Part model, mm, in its own coordinate system. Face numbers are marked on the shaded views. A direction names the side the tool comes from. Give positions to 0.01 mm unless a question says otherwise; leave off trailing zeros. Write each loop counter-clockwise with the first axis right and the second up, starting at its lowest first coordinate (ties: lowest second). Pieces come first, ordered by that corner, then holes. Notation, with made-up numbers: M 2.5,66 L 58.5,66 A34 ccw 58.5,104 Z; hole C 48.5,-16.5 d4. An arc over 180 degrees is marked long. Use a Markdown table: item, result.
```python
from build123d import *
from build123d.topology import SkipClean

# Parameters (mm, degrees)
SKETCH1_R           = 1.1
BOSS_EXTRUDE1_DEPTH = 1.5
SKETCH2_R           = 2.5
BOSS_EXTRUDE2_DEPTH = 1
BOSS_EXTRUDE3_DEPTH = 4
BOSS_EXTRUDE4_START = 5
SKETCH4_W           = 6
SKETCH4_H           = 14
SKETCH4_R           = 1.1
BOSS_EXTRUDE4_DEPTH = 5
FILLET4_R           = 3
FILLET1_R           = 0.5
SKETCH5_R           = 1.75
CUT_EXTRUDE1_DEPTH  = 4
FILLET3_R           = 2


with BuildPart() as part:
    # Sketch1 → Boss-Extrude1 (new body)
    with BuildSketch(Plane.XY):
        with BuildLine():
            Line((-17, 7), (0, 7))
            ThreePointArc((0, 7), (7, 0), (0, -7))
            Line((0, -7), (-17, -7))
            Line((-17, -7), (-17, 7))
        make_face()
        with Locations((-14, 3.5)):
            Circle(SKETCH1_R, mode=Mode.SUBTRACT)
        with Locations(Location((-14, -3.5, 0), (0, 0, 180))):
            Circle(SKETCH1_R, mode=Mode.SUBTRACT)
    extrude(amount=BOSS_EXTRUDE1_DEPTH)

    # Sketch2 → Boss-Extrude2 (add)
    with BuildSketch(Plane(origin=(0, 0, 0), x_dir=(-1, 0, 0), z_dir=(0, 0, -1))):
        Circle(SKETCH2_R)
    extrude(amount=BOSS_EXTRUDE2_DEPTH)

    # Sketch3 → Boss-Extrude3 (add)
    with BuildSketch(Plane(origin=(0, 0, -1), x_dir=(-1, 0, 0), z_dir=(0, 0, -1))):
        with BuildLine():
            Line((1.13862177, 1.394109201), (1.13862177, -1.394109201))
            ThreePointArc((1.13862177, -1.394109201), (-1.8, 0), (1.13862177, 1.394109201))
        make_face()
    extrude(amount=BOSS_EXTRUDE3_DEPTH)

    # Sketch4 → Boss-Extrude4 (add)
    with SkipClean():  # the faces are left unmerged after this step: merging them gives an invalid solid
        with BuildSketch(Plane(origin=(0, 0, 0), x_dir=(-1, 0, 0), z_dir=(0, 0, -1)).offset(BOSS_EXTRUDE4_START)):
            with Locations((14, 0)):
                Rectangle(SKETCH4_W, SKETCH4_H)
            with Locations((14, 3.5)):
                Circle(SKETCH4_R, mode=Mode.SUBTRACT)
            with Locations((14, -3.5)):
                Circle(SKETCH4_R, mode=Mode.SUBTRACT)
        extrude(amount=-BOSS_EXTRUDE4_DEPTH)

    # Fillet4
    fillet4_edges = [part.edges().sort_by_distance(p)[0] for p in [
        (-17, -7, -2.5),
        (-17, 7, -2.5),
    ]]
    fillet(fillet4_edges, radius=FILLET4_R)

    # Fillet1
    fillet1_edges = [part.edges().sort_by_distance(p)[0] for p in [
        (7, 0, 1.5),
        (-17, 0, 1.5),
        (-7, -7, 1.5),
        (-16.121320344, -6.121320344, 1.5),
        (-16.121320344, 6.121320344, 1.5),
        (-7, 7, 1.5),
    ]]
    fillet(fillet1_edges, radius=FILLET1_R)

    # Sketch5 → Cut-Extrude1 (cut)
    with BuildSketch(Plane.XY.offset(1.5)):
        with Locations((-14, 3.5)):
            Circle(SKETCH5_R)
        with Locations((-14, -3.5)):
            Circle(SKETCH5_R)
    extrude(amount=-CUT_EXTRUDE1_DEPTH, mode=Mode.SUBTRACT)

    # Fillet3
    fillet3_edges = [part.edges().sort_by_distance(p)[0] for p in [
        (-11, 0, 0),
    ]]
    fillet(fillet3_edges, radius=FILLET3_R)


solid = part.part
```
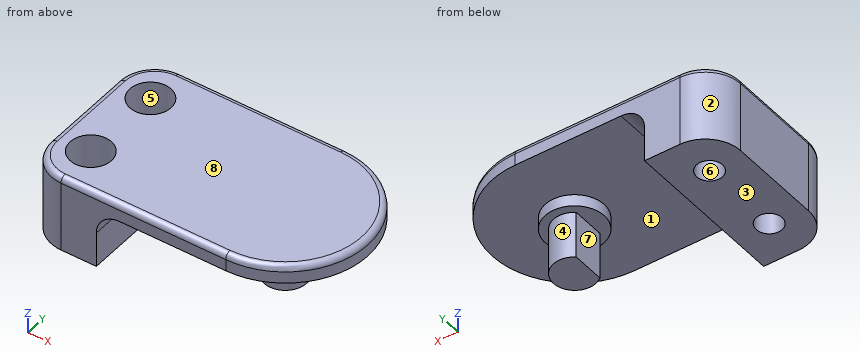
1. Cut at A-A, the plane z = -4. Give the cut face in (x, y), then the cut area to 3 significant figures.
Findings below:
| item | result |
|---|---|
| outline | M -17,-4 A3 ccw -14,-7 L -11,-7 L -11,7 L -14,7 A3 ccw -17,4 Z; M -1.14,-1.39 A1.8 ccw long -1.14,1.39 Z; hole C -14,-3.5 d2.2; hole C -14,3.5 d2.2 |
| area | 81.4 mm2 |
2. Drop flat-ended pins along their axis: P1, Ø2, axis at x = -4, z = -1.5, coming from the -Y side; P2, Ø1.5, axis at y = 3, z = -3.5, coming from the +X side; P3, Ø2.5, axis at x = -14, y = 3.5, coming from the +Z side; P4, Ø1.5, axis at y = 1, z = -2.5, coming from the +X side. Give the stop position or say it passes through.
Findings below:
| item | result |
|---|---|
| P1 | through |
| P2 | x = -11 |
| P3 | z = -2.5 |
| P4 | x = 1.78 |
3. Two-plate mould, pull along X, no slides. Class the marked faces 1, 2 and 3: released by +X, released by -X, zero draft, split by the parting line, or undercut.
Findings below:
| item | result |
|---|---|
| face 1 | undercut |
| face 2 | released by -X |
| face 3 | zero draft |
4. Drill centre lines: L1, parallel to Y at x = -14, z = -0.7; L2, parallel to Y at x = -14, z = -4; L3, parallel to X at y = -3, z = -4.5. Where is each one in solid material? Low to high.
Findings below:
| item | result |
|---|---|
| L1 | -7 to -5.25, -1.75 to 1.75, 5.25 to 7 |
| L2 | -7 to -4.6, -2.4 to 2.4, 4.6 to 7 |
| L3 | -17 to -14.98, -13.02 to -11 |
5. Tool access for the marked faces 4, 5, 6, 7 and 8: list every direction of +Z, -Z, +X, -X, +Y, -Y with a clear straight run to the whole face (end or side of a thin tool).
Findings below:
| item | result |
|---|---|
| face 4 | -Z |
| face 5 | +Z |
| face 6 | +Z, -Z |
| face 7 | -Z, +Y, -Y |
| face 8 | +Z, +X, -X, +Y, -Y |
6. Cut at B-B, the plane z = 0.25. Give the cut face in (x, y).
Findings below:
| item | result |
|---|---|
| outline | M -17,-4 A3 ccw -14,-7 L 0,-7 A7 ccw 0,7 L -14,7 A3 ccw -17,4 Z; hole C -14,-3.5 d3.5; hole C -14,3.5 d3.5 |
7. Cut at D-D, the plane z = -1.75. Give the cut face in (x, y).
Findings below:
| item | result |
|---|---|
| outline | M -17,-4 A3 ccw -14,-7 L -10.98,-7 L -10.98,7 L -14,7 A3 ccw -17,4 Z; M -1.14,-1.39 A1.8 ccw long -1.14,1.39 Z; hole C -14,-3.5 d3.5; hole C -14,3.5 d3.5 |
8. Cut at C-C, the plane y = 0. Give the cut face in (x, z), then the cut area to 3 significant figures.
Findings below:
| item | result |
|---|---|
| outline | M -17,-5 L -11,-5 L -11,-2 A2 cw -9,0 L -2.5,0 L -2.5,-1 L -1.14,-1 L -1.14,-5 L 1.8,-5 L 1.8,-1 L 2.5,-1 L 2.5,0 L 7,0 L 7,1 A0.5 ccw 6.5,1.5 L -16.5,1.5 A0.5 ccw -17,1 Z |
| area | 83.5 mm2 |
